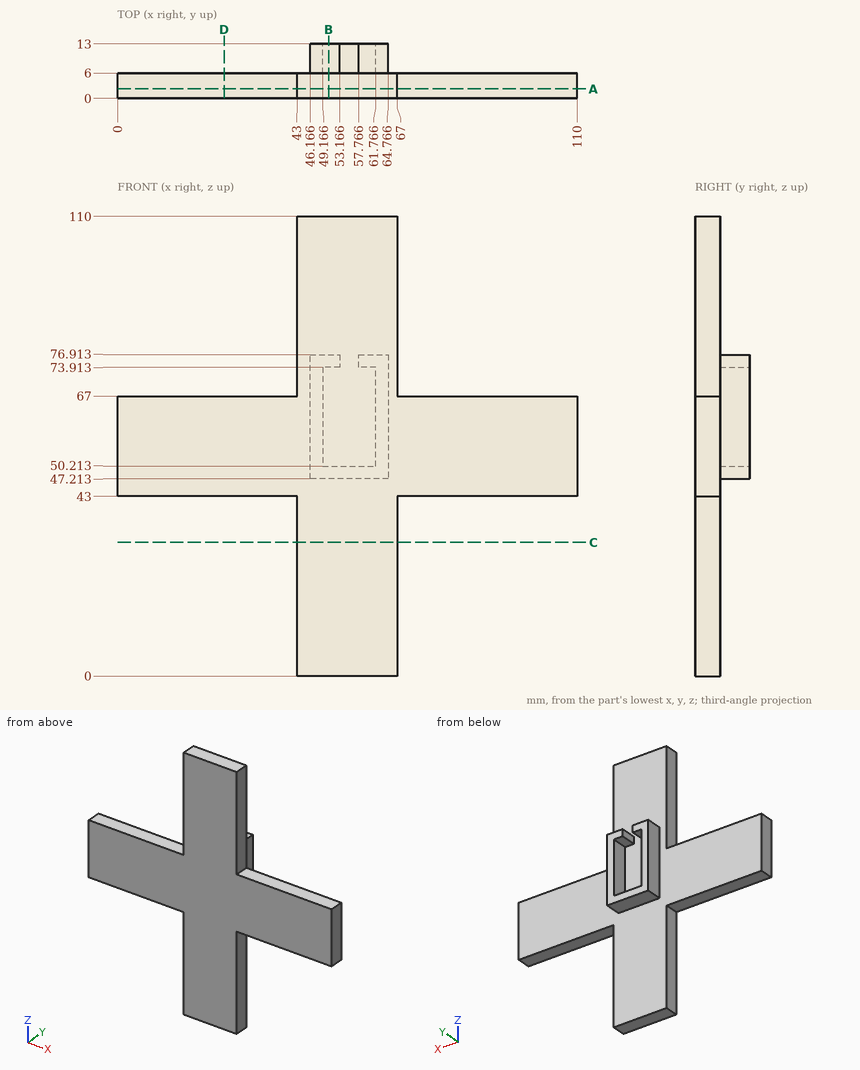
Design review of the part shown in the three views and the two pictorial views. Dimensions are in mm from the part's minimum x, y and z. Give positions to 0.01 mm unless a question says otherwise; leave off trailing zeros. Loops run counter-clockwise (first coordinate to the right, second up) from the corner with the lowest first, then second, coordinate; pieces in that order, holes last. Notation, with made-up numbers: M 59.25,11 L 73.25,11 A28 ccw 73.25,36 Z; hole C 86.5,-17 d10. An arc over 180 degrees is marked long. Answer as a JSON object with one key per item and string values. Group by question number.
Q1. Add section C-C on z = 32. Give the boundary of the cut face in (x, y), and give its area (3 significant figures).
Q2. For probe 1 along Y at (x, z) = (5.5, 43.5); probe 2 along X at (y, z) = (1, 74.5), list the stretches that pass through material, from the lowest coordinate up. Write a range as [from, to].
Q3. Insertion check: P1, Ø10, axis at x = 76, z = 47, coming from the +Y side; P2, Ø3, axis at x = 92.5, y = 6, coming from the +Z side; P3, Ø1.8, axis at x = 82.5, y = 2.5, coming from the -Z side. Each pin has a flat end and moves straight along its axis. Give the tip position at first contact, or say it passes through.
Q4. Add section B-B on x = 50.5. Give the boundary of the cut face in (y, z).
Q5. Add section A-A on y = 2.25. Give the boundary of the cut face in (x, z), and give its area (3 significant figures).
Q6. Add section D-D on x = 25.5. Give the boundary of the cut face in (y, z), and give its area (3 significant figures).
Checked values:
{
 "1": {"outline": "M 43,0 L 67,0 L 67,6 L 43,6 Z", "area": "144 mm²"},
 "2": {"probe 1": "[0, 6]", "probe 2": "[43, 67]"},
 "3": {"P1": "y = 6", "P2": "z = 67", "P3": "z = 43"},
 "4": {"outline": "M 0,0 L 6,0 L 6,47.21 L 13,47.21 L 13,50.21 L 6,50.21 L 6,73.91 L 13,73.91 L 13,76.91 L 6,76.91 L 6,110 L 0,110 Z"},
 "5": {"outline": "M 0,43 L 43,43 L 43,0 L 67,0 L 67,43 L 110,43 L 110,67 L 67,67 L 67,110 L 43,110 L 43,67 L 0,67 Z", "area": "4,700 mm²"},
 "6": {"outline": "M 0,43 L 6,43 L 6,67 L 0,67 Z", "area": "144 mm²"}
}
